from build123d import *

# Parameters (mm, degrees)
BOSS_EXTRUDE1_DEPTH       = 1
BOSS_EXTRUDE1_DEPTH_BACK  = 2
SKETCH1_W                 = 60
SKETCH1_H                 = 90
SKETCH2_R                 = 2
BOSS_EXTRUDE2_DEPTH       = 3.5
SKETCH3_R                 = 3.5
BOSS_EXTRUDE3_DEPTH       = 2.5
CHAMFER1_SIZE             = 1
BOSS_EXTRUDE5_START       = -42
BOSS_EXTRUDE5_OUTLINE_W   = 60
BOSS_EXTRUDE5_OUTLINE_H   = 90
BOSS_EXTRUDE5_DEPTH       = 40
BOSS_EXTRUDE5_START_2     = 11.244510856
BOSS_EXTRUDE5_2_OUTLINE_W = 68
BOSS_EXTRUDE5_2_OUTLINE_H = 101
BOSS_EXTRUDE5_2_DEPTH     = 38.755489144
BOSS_EXTRUDE6_REACH       = 116.704
CHAMFER2_SIZE             = 3
FILLET1_R                 = 5


with BuildPart() as part:
    # Sketch1 → Boss-Extrude1 (new, two sides: drawn at the far end of the back side and taken through both)
    with BuildSketch(Plane(origin=(0, 0, 0), x_dir=(1, 0, 0), z_dir=(0, 1, 0)).offset(-BOSS_EXTRUDE1_DEPTH_BACK)):
        with Locations((30, -45)):
            Rectangle(SKETCH1_W, SKETCH1_H)
    extrude(amount=BOSS_EXTRUDE1_DEPTH + BOSS_EXTRUDE1_DEPTH_BACK)

    # Sketch2 → Boss-Extrude2 (add)
    with BuildSketch(Plane(origin=(0, 1, 0), x_dir=(1, 0, 0), z_dir=(0, 1, 0))):
        with Locations(Location((30, -23, 0), (0, 0, 90))):
            Circle(SKETCH2_R)
        with Locations(Location((30, -67, 0), (0, 0, 90))):
            Circle(SKETCH2_R)
    extrude(amount=BOSS_EXTRUDE2_DEPTH)

    # Sketch3 → Boss-Extrude3 (add)
    with BuildSketch(Plane(origin=(0, 4.5, 0), x_dir=(1, 0, 0), z_dir=(0, 1, 0))):
        with Locations(Location((30, -23, 0), (0, 0, 270))):
            Circle(SKETCH3_R)
        with Locations(Location((30, -67, 0), (0, 0, 270))):
            Circle(SKETCH3_R)
    extrude(amount=BOSS_EXTRUDE3_DEPTH)

    # Chamfer1
    chamfer1_edges = [part.edges().sort_by_distance(p)[0] for p in [
        (30, 4.5, 19.5),
        (30, 4.5, 63.5),
    ]]
    chamfer(chamfer1_edges, length=CHAMFER1_SIZE)

    # Boss-Extrude5: read off the stored shape, not the designer's step
    # Boss-Extrude5 outline → Boss-Extrude5 (add)
    with BuildSketch(Plane(origin=(0, 0, 0), x_dir=(1, 0, 0), z_dir=(0, 1, 0)).offset(BOSS_EXTRUDE5_START)):
        with Locations((30, -45)):
            Rectangle(BOSS_EXTRUDE5_OUTLINE_W, BOSS_EXTRUDE5_OUTLINE_H)
    extrude(amount=BOSS_EXTRUDE5_DEPTH)

    # Boss-Extrude5 2 outline → Boss-Extrude5 2 (cut)
    with BuildSketch(Plane(origin=(0, 0, 0), x_dir=(0.9877295966495896, 0.14815943949743834, 0.049386479832479395), z_dir=(0.15617376188860593, -0.9370425713316366, -0.31234752377721187)).offset(BOSS_EXTRUDE5_START_2)):
        with Locations((26, 49.5)):
            Rectangle(BOSS_EXTRUDE5_2_OUTLINE_W, BOSS_EXTRUDE5_2_OUTLINE_H)
    extrude(amount=BOSS_EXTRUDE5_2_DEPTH, mode=Mode.SUBTRACT)

    # Boss-Extrude6: up to this plane
    boss_extrude6_end = Plane(origin=(0, -2, 0), z_dir=(0, 0, -1))
    # Sketch11 → Boss-Extrude6 (add, up to the surface)
    with BuildSketch(Plane(origin=(5.05471325, -30.328279499, 93.512195122), x_dir=(-0.9986694407655652, -0.011316895385518406, 0.05031178748391653), z_dir=(-0.05134961659630974, 0.3080976995778579, -0.9499679070317293)), mode=Mode.PRIVATE) as boss_extrude6_sk1:
        Polygon((-20.078587448, -8.116309156), (-25.01329722, -7.310927591), (-27.026751132, -19.647702021), (-19.131215496, -20.936312525), (-18.084219462, -14.521189821), (-21.045045326, -14.037960882), align=None)
    boss_extrude6_tool1 = split(extrude(boss_extrude6_sk1.sketch, amount=BOSS_EXTRUDE6_REACH, mode=Mode.PRIVATE), bisect_by=boss_extrude6_end, keep=Keep.BOTH, mode=Mode.PRIVATE)
    add(boss_extrude6_tool1.solids().sort_by_distance((27.683241, -44.092393, 87.824995))[0])
    # Sketch11 → Boss-Extrude6 (add, up to the surface)
    with BuildSketch(Plane(origin=(5.05471325, -30.328279499, 93.512195122), x_dir=(-0.9986694407655652, -0.011316895385518406, 0.05031178748391653), z_dir=(-0.05134961659630974, 0.3080976995778579, -0.9499679070317293)), mode=Mode.PRIVATE) as boss_extrude6_sk2:
        Polygon((-27.026751132, -19.647702021), (-25.01329722, -7.310927591), (-29.948006992, -6.505546026), (-30.91446487, -12.427197753), (-33.875290733, -11.943968814), (-34.922286767, -18.359091518), align=None)
    boss_extrude6_tool2 = split(extrude(boss_extrude6_sk2.sketch, amount=BOSS_EXTRUDE6_REACH, mode=Mode.PRIVATE), bisect_by=boss_extrude6_end, keep=Keep.BOTH, mode=Mode.PRIVATE)
    add(boss_extrude6_tool2.solids().sort_by_distance((34.491765, -42.957639, 87.824995))[0])

    # Chamfer2
    chamfer2_edges = [part.edges().sort_by_distance(p)[0] for p in [
        (21.734111013, -36.066766318, 43.047827976),
        (37.516413794, -33.436382521, 43.047827976),
    ]]
    chamfer(chamfer2_edges, length=CHAMFER2_SIZE)

    # Fillet1
    fillet1_edges = [part.edges().sort_by_distance(p)[0] for p in [
        (0, -5.5, 0),
        (60, -0.5, 0),
        (60, -15.5, 90),
        (0, -20.5, 90),
    ]]
    fillet(fillet1_edges, radius=FILLET1_R)


solid = part.part
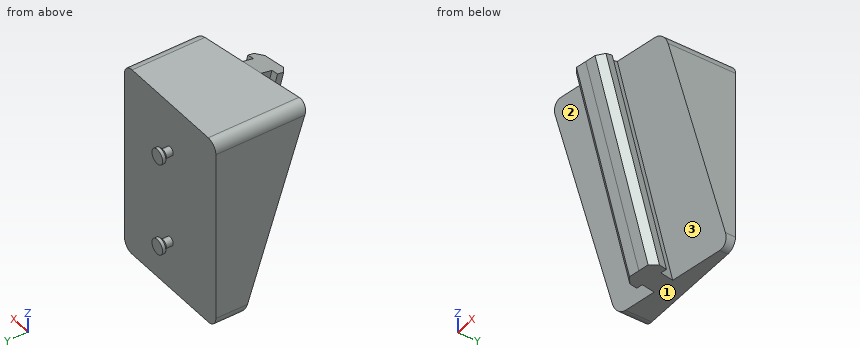
The listing builds one solid part. Answer for the finished solid, in the listing's coordinates (mm). Face numbers are marked on the shaded views. Coordinates: 2 decimals unless noted, no trailing zeros. Write each loop counter-clockwise with the first axis right and the second up, starting at its lowest first coordinate (ties: lowest second). Pieces come first, ordered by that corner, then holes. Notation, with made-up numbers: M 24.5,-32 L 52.5,-32 A17 cw 52.5,-13 Z; hole C -29.75,34.5 d4. An arc over 180 degrees is marked long. Write each question's results on one line, items separated by ' | '.
Item 1: Given P1, Ø8, axis at x = 53, z = 34.5, coming from the +Y side; P2, Ø1, axis at x = 37.5, z = 15, coming from the -Y side; P3, Ø4, axis at x = 29, z = 23.5, coming from the -Y side, each flat-ended and moving along its own axis, determine where each tip first touches the part or whether it passes through.
Answer below:
P1: y = 1 | P2: y = -10.94 | P3: y = -29.09
Item 2: The part is cut by section D-D on z = 67. Determine the outline of the cut face in (x, y), and give its area (3 significant figures).
Answer below:
outline: M 0,-34.33 L 23.82,-30.36 L 24.86,-36.59 L 21.9,-37.09 L 22.51,-40.72 L 25.99,-43.34 L 35.85,-41.7 L 38.29,-38.09 L 37.69,-34.46 L 34.73,-34.95 L 33.69,-28.72 L 60,-24.33 L 60,1 L 32,1 L 32,4.5 L 32.5,4.5 L 33.5,5.5 L 33.5,7 L 26.5,7 L 26.5,5.5 L 27.5,4.5 L 28,4.5 L 28,1 L 0,1 Z | area: 2,010 mm2
Item 3: For a pull along X with two mould halves and no side action, classify the marked faces 1, 2 and 3 as released by +X, released by -X, zero draft, split by the parting line, or undercut.
Answer below:
face 1: zero draft | face 2: undercut | face 3: released by +X
Item 4: Consider probe 1 along Y at (x, z) = (48, 44); probe 2 along Y at (x, z) = (45.5, 17.5); probe 3 along X at (y, z) = (-27, 33). Determine where each line is inside the solid, lowest interval first. Write a range as [from, to].
Answer below:
probe 1: [-18.67, 1] | probe 2: [-10.25, 1] | probe 3: [20.22, 36.44]
Item 5: The part is cut by section A-A on z = 35. Determine the outline of the cut face in (x, y), and give its area (3 significant figures).
Answer below:
outline: M 0,-23.67 L 22.1,-19.98 L 23.13,-26.21 L 20.17,-26.71 L 20.78,-30.34 L 24.26,-32.96 L 34.12,-31.32 L 36.56,-27.71 L 35.96,-24.08 L 33,-24.57 L 31.96,-18.34 L 60,-13.67 L 60,1 L 0,1 Z | area: 1,340 mm2
Item 6: The part is cut by section C-C on x = 41. Determine the outline of the cut face in (y, z), and give its area (4 significant figures).
Answer below:
outline: M -35.17,90 L -5.17,0 L 1,0 L 1,90 Z | area: 1,905 mm2
Item 7: The part is cut by section B-B on y = -34. Determine the outline of the cut face in (x, z).
Answer below:
outline: M 0,66 L 24.43,78.22 L 24.43,59.01 L 21.39,57.49 L 21.39,46.28 L 24.43,38.2 L 34.57,43.26 L 37.61,54.39 L 37.61,65.6 L 34.57,64.08 L 34.57,83.28 L 48,90 L 5,90 A5 ccw 0,85 Z
